```python
from build123d import *

# Parameters (mm, degrees)
SKETCH1_W                                    = 165.1
SKETCH1_H                                    = 165.1
SKETCH1_R                                    = 13.096875
SKETCH1_R_2                                  = 1.5875
BOSS_EXTRUDE1_DEPTH                          = 6.35
SKETCH3_R                                    = 15.875
CUT_EXTRUDE1_DEPTH                           = 4.7625
CSK_FOR_1_4_FLAT_HEAD_SOCKET_CAP_SCR_2_COUNT = 2
CSK_FOR_1_4_FLAT_HEAD_SOCKET_CAP_SCR_2_PITCH = 81.129190467
CSK_FOR_1_4_FLAT_HEAD_SOCKET_CAP_SCR_3_COUNT = 2
CSK_FOR_1_4_FLAT_HEAD_SOCKET_CAP_SCR_3_PITCH = 68.88094119
FILLET1_R                                    = 6.35
F_10_CLEARANCE_HOLE1_D                       = 5.1054
F_10_24_TAPPED_HOLE1_D                       = 3.7973
F_10_24_TAPPED_HOLE1_DEPTH                   = 16.002
F_10_24_TAPPED_HOLE1_TIP                     = 1.140824014
F_10_CLEARANCE_HOLE2_D                       = 5.1054
SKETCH16_R                                   = 19.446875
SKETCH16_R_2                                 = 9.7282
SKETCH16_R_3                                 = 8.24865
CUT_EXTRUDE2_DEPTH                           = 3.175
FILLET2_R                                    = 3.175
F_10_32_TAPPED_HOLE1_D                       = 4.0386


with BuildPart() as part:
    # Sketch1 → Boss-Extrude1 (new body)
    with BuildSketch(Plane(origin=(0, 0, 0), x_dir=(1, 0, 0), z_dir=(0, 1, 0))):
        Rectangle(SKETCH1_W, SKETCH1_H)
        with Locations((-19.05, -12.7)):
            Circle(SKETCH1_R, mode=Mode.SUBTRACT)
        with Locations((23.8125, -12.7)):
            Circle(SKETCH1_R_2, mode=Mode.SUBTRACT)
    extrude(amount=BOSS_EXTRUDE1_DEPTH)

    # Sketch3 → Cut-Extrude1 (cut)
    with BuildSketch(Plane.XZ.offset(-6.35)):
        with Locations((-19.05, 12.7)):
            Circle(SKETCH3_R)
    extrude(amount=CUT_EXTRUDE1_DEPTH, mode=Mode.SUBTRACT)

    # Sketch8 → CSK for 1/4 Flat Head Socket Cap Screw1 (revolve, cut)
    with BuildSketch(Plane(origin=(-62.992, 6.35, 20.574), x_dir=(0, 0, 1), z_dir=(1, 0, 0))):
        Polygon((0, 0), (0, 6.35), (3.3782, 6.35), (3.3782, 3.871564875), (6.7437, 0), align=None)
    csk_for_1_4_flat_head_socket_cap_screw1 = revolve(axis=Axis((-62.992, 12.7, 20.574), (0, -1, 0)), mode=Mode.SUBTRACT)

    # CSK for 1_4 Flat Head Socket Cap Scr 2: CSK for 1/4 Flat Head Socket Cap Screw1 ×2
    with Locations(*[Vector(0.925467142, 0, -0.378827889) * (i * CSK_FOR_1_4_FLAT_HEAD_SOCKET_CAP_SCR_2_PITCH) for i in range(1, CSK_FOR_1_4_FLAT_HEAD_SOCKET_CAP_SCR_2_COUNT)]):
        add(csk_for_1_4_flat_head_socket_cap_screw1, mode=Mode.SUBTRACT)

    # CSK for 1_4 Flat Head Socket Cap Scr 3: CSK for 1/4 Flat Head Socket Cap Screw1 ×2
    with Locations(*[Vector(0.862142691, 0, 0.506665551) * (i * CSK_FOR_1_4_FLAT_HEAD_SOCKET_CAP_SCR_3_PITCH) for i in range(1, CSK_FOR_1_4_FLAT_HEAD_SOCKET_CAP_SCR_3_COUNT)]):
        add(csk_for_1_4_flat_head_socket_cap_screw1, mode=Mode.SUBTRACT)

    # Fillet1
    fillet1_edges = [part.edges().sort_by_distance(p)[0] for p in [
        (-82.55, 3.175, -82.55),
        (82.55, 3.175, -82.55),
        (82.55, 3.175, 82.55),
        (-82.55, 3.175, 82.55),
    ]]
    fillet(fillet1_edges, radius=FILLET1_R)

    # #10 Clearance Hole1 (through all)
    with Locations(Plane(origin=(0, 6.35, 0), x_dir=(1, 0, 0), z_dir=(0, 1, 0))):
        with Locations((-76.2, -76.2), (-76.2, 76.2), (76.2, 76.2), (76.2, -76.2), (0, 76.2), (0, -76.2), (-76.2, 0), (76.2, 0)):
            Hole(F_10_CLEARANCE_HOLE1_D / 2)

    # #10-24 Tapped Hole1
    with Locations(Plane(origin=(0, 6.35, 0), x_dir=(1, 0, 0), z_dir=(0, 1, 0))):
        with Locations((23.8125, -12.7), (-49.358364409, -43.008364409), (-19.05, 30.1625), (-19.05, -12.7)):
            Hole(F_10_24_TAPPED_HOLE1_D / 2, depth=F_10_24_TAPPED_HOLE1_DEPTH)
            with Locations((0, 0, -(F_10_24_TAPPED_HOLE1_DEPTH + F_10_24_TAPPED_HOLE1_TIP / 2))):  # 118° drill point
                Cone(0, F_10_24_TAPPED_HOLE1_D / 2, F_10_24_TAPPED_HOLE1_TIP, mode=Mode.SUBTRACT)

    # #10 Clearance Hole2 (through all)
    with Locations(Plane(origin=(0, 6.35, 0), x_dir=(1, 0, 0), z_dir=(0, 1, 0))):
        with Locations((23.8125, 30.1625), (4.7625, 30.1625)):
            Hole(F_10_CLEARANCE_HOLE2_D / 2)

    # Sketch16 → Cut-Extrude2 (cut)
    with BuildSketch(Plane.XZ):
        with BuildLine():
            Line((69.85, -69.85), (-69.85, -69.85))
            Line((-69.85, -69.85), (-69.85, 13.674310787))
            ThreePointArc((-69.85, 13.674310787), (-53.2638, 20.574), (-69.85, 27.473689213))
            Line((-69.85, 27.473689213), (-69.85, 69.85))
            Line((-69.85, 69.85), (69.85, 69.85))
            Line((69.85, 69.85), (69.85, -69.85))
        make_face()
        with Locations((-19.05, 12.7)):
            Circle(SKETCH16_R, mode=Mode.SUBTRACT)
        with Locations((-3.6068, 55.4736)):
            Circle(SKETCH16_R_2, mode=Mode.SUBTRACT)
        with Locations((23.8125, 12.7)):
            Circle(SKETCH16_R_3, mode=Mode.SUBTRACT)
        with Locations((-19.05, -30.1625)):
            Circle(SKETCH16_R_3, mode=Mode.SUBTRACT)
        with Locations((-49.358364409, 43.008364409)):
            Circle(SKETCH16_R_3, mode=Mode.SUBTRACT)
        with BuildLine():
            ThreePointArc((20.819224907, -14.454821414), (11.727367105, -0.438576115), (3.70620807, -15.093882946))
            ThreePointArc((3.70620807, -15.093882946), (4.113625171, -19.033669627), (1.400289966, -21.919101976))
            ThreePointArc((1.400289966, -21.919101976), (-2.687905399, -35.035848611), (10.967913569, -36.546143923))
            ThreePointArc((10.967913569, -36.546143923), (14.2875, -35.198574694), (17.607086431, -36.546143923))
            ThreePointArc((17.607086431, -36.546143923), (31.895360473, -33.894179765), (24.646386862, -21.298939768))
            ThreePointArc((24.646386862, -21.298939768), (20.935730068, -18.881787262), (20.819224907, -14.454821414))
        make_face(mode=Mode.SUBTRACT)
    extrude(amount=-CUT_EXTRUDE2_DEPTH, mode=Mode.SUBTRACT)

    # Fillet2
    fillet2_edges = [part.edges().sort_by_distance(p)[0] for p in [
        (-69.85, 1.5875, 13.674310787),
        (-69.85, 1.5875, 27.473689213),
        (-69.85, 1.5875, 69.85),
        (69.85, 1.5875, 69.85),
        (69.85, 1.5875, -69.85),
        (-69.85, 1.5875, -69.85),
    ]]
    fillet(fillet2_edges, radius=FILLET2_R)

    # #10-32 Tapped Hole1 (through all)
    with Locations(Plane(origin=(0, 6.35, 0), x_dir=(1, 0, 0), z_dir=(0, 1, 0))):
        with Locations((58.7375, 44.45), (-58.7375, 44.45)):
            Hole(F_10_32_TAPPED_HOLE1_D / 2)


solid = part.part
```
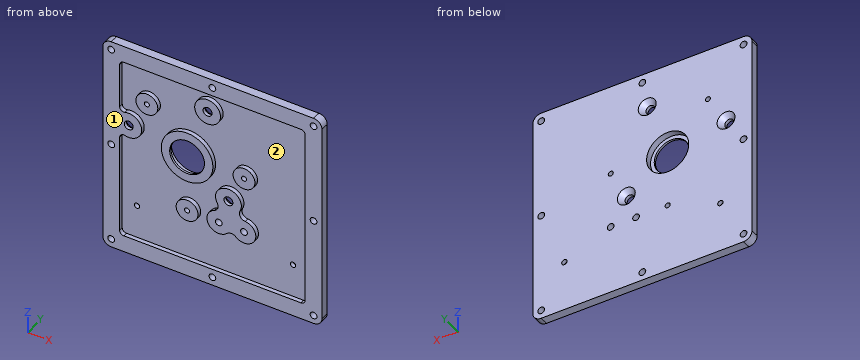
For this review, take the finished solid that the model builds, in its own axes (mm). Face numbers are marked on the shaded views. Round coordinates to 2 decimals unless told otherwise and drop trailing zeros. Write each loop counter-clockwise with the first axis right and the second up, starting at its lowest first coordinate (ties: lowest second). Pieces come first, ordered by that corner, then holes. Notation, with made-up numbers: M -10,11.5 L 3,11.5 A9 ccw 3,18.5 Z; hole C 75,82.5 d6. An arc over 180 degrees is marked long. One line per item, written item: value. Start each with the question number.
(1) Wall thickness on line 1 (X direction, y = 3.75, z = -76.2); line 2 (Z direction, x = -63, y = 0.5); line 3 (Z direction, x = -19.05, y = 4.5) (3 decimals): over which ranges is each line inside the solid? List them lowest first.
(2) The part is to be moulded in two halves that separate along Z. For the marked faces 1 and 2, say which applies: released by +Z, released by -Z, zero draft, split by the parting line, or undercut.
(3) We need section D-D (x = 46.5). Give the boundary of the cut face in (y, z) (3 decimals).
(4) We need section B-B (z = -10.16). Give the boundary of the cut face in (x, y) (3 decimals).
(5) Insertion check: pin 1 (11 mm diameter, centred on x = -3.61, z = 55.47, fed in from +Y); pin 2 (12 mm diameter, centred on x = 49, z = -18.5, fed in from -Y) (3 decimals); pin 3 (4 mm diameter, centred on x = -62.992, z = 20.574, fed in from +Y). Each pin has a flat end and moves straight along its axis. Give the tip position at first contact, or say it passes through.
(6) We need section A-A (x = -19.05). Count the separate pieces of the cut face and the enclosed holes in it, and give its area (3 significant figures).
Result:
1. line 1: -82.55 to -78.75, -73.65 to -2.55, 2.55 to 73.65, 78.75 to 82.55
1. line 2: -82.55 to -69.85, 10.85 to 17.2, 23.95 to 30.3, 69.85 to 82.55
1. line 3: -82.55 to -32.061, -28.264 to -3.175, 28.575 to 82.55
2. face 1: zero draft
2. face 2: undercut
3. outline: M 0,-82.55 L 6.35,-82.55 L 6.35,82.55 L 0,82.55 L 0,69.85 L 3.175,69.85 L 3.175,-69.85 L 0,-69.85 Z
4. outline: M -82.55,0 L -69.85,0 L -69.85,3.175 L 2.362,3.175 L 2.362,0 L 8.712,0 L 8.712,2.478 L 5.347,6.35 L -82.55,6.35 Z; M 15.469,0 L 21.819,0 L 21.819,3.175 L 69.85,3.175 L 69.85,0 L 82.55,0 L 82.55,6.35 L 18.834,6.35 L 15.469,2.478 Z
5. pin 1: y = 4.92
5. pin 2: y = 3.175
5. pin 3: through
6. separate pieces: 3
6. enclosed holes: 0
6. area: 564 mm²
